Can you work these out from the model? Positions are in its coordinate system, mm. Face numbers are marked on the shaded views. A direction names the side the tool comes from. Round coordinates to 2 decimals unless told otherwise and drop trailing zeros. Loops run counter-clockwise (first coordinate to the right, second up) from the corner with the lowest first, then second, coordinate; pieces in that order, holes last. Notation, with made-up numbers: (27.5, 64) -> (54.5, 64) arc R6 ccw to (54.5, 68) -> close; hole circle Ø10 at (-24, 50). An arc over 180 degrees is marked (long way). Answer as a JSON object with one key per item and string values.
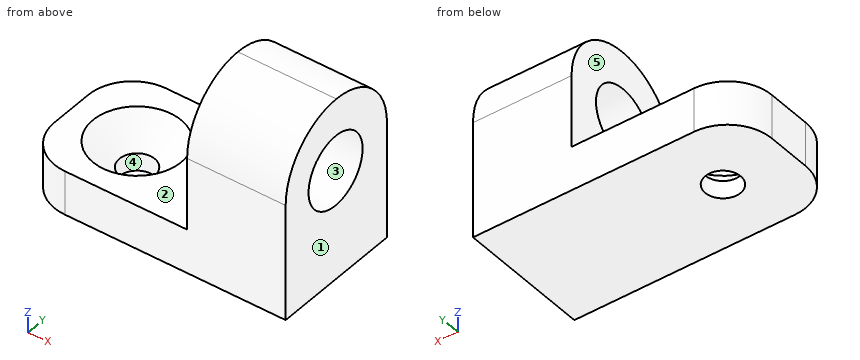
```python
from build123d import *

# Parameters (mm, degrees)
F0_W     = 18.8419777411
F0_H     = 15
F0_R     = 2
F0_W_2   = 11.1580222589
F1_DEPTH = 5
F2_SIZE  = 3
F3_DEPTH = 20.7
F4_R     = 4
F5_DEPTH = 55.3
F6_R     = 7.49999
F7_R     = 5


# Not quite as in the source:
# - a fillet or chamfer is up to 0.001 mm smaller than in the source, because OpenCascade refuses the exact size


with BuildPart() as f1:
    # F0 (on Top) → F1 (new body)
    with BuildSketch(Plane.XY):
        with Locations((9.4734227529, 0.1149109378)):
            Rectangle(F0_W, F0_H)
        with Locations((7.5819236226, 0)):
            Circle(F0_R, mode=Mode.SUBTRACT)
        with Locations((24.4734227529, 0.1149109378)):
            Rectangle(F0_W_2, F0_H)
    extrude(amount=F1_DEPTH)

    # F2
    f2_edges = [f1.edges().sort_by_distance(p)[0] for p in [
        (5.581924, 0, 5),
    ]]
    chamfer(f2_edges, length=F2_SIZE)

    # F0 (on Top) → F3 (join)
    with BuildSketch(Plane.XY):
        with Locations((24.4734227529, 0.1149109378)):
            Rectangle(F0_W_2, F0_H)
    extrude(amount=F3_DEPTH)

    # F4 (on Right) → F5 (cut)
    with BuildSketch(Plane.YZ):
        with Locations((0, 12.5060472637)):
            Circle(F4_R)
    extrude(amount=F5_DEPTH, mode=Mode.SUBTRACT)

    # F6 (radius 7.5 in the source; OpenCascade refuses exactly that, so slightly less here)
    f6_edges = [f1.edges().sort_by_distance(p)[0] for p in [
        (24.473423, -7.385089, 20.7),
        (24.473423, 7.614911, 20.7),
    ]]
    fillet(f6_edges, radius=F6_R)

    # F7
    f7_edges = [f1.edges().sort_by_distance(p)[0] for p in [
        (0.052434, -7.385089, 2.5),
        (0.052434, 7.614911, 2.5),
    ]]
    fillet(f7_edges, radius=F7_R)


solid = f1.part
```
Q1. I'm going to push a flat-ended pin straight in: pin 1 (4 mm diameter, centred on x = 17.5, y = 1, fed in from +Z). Where does the tip first touch, or does it pass through?
Determined:
{"pin 1": "z = 20.7"}
Q2. I want a section at D-D, the plane y = -6.25. Write out the boundary of the cut face in (x, z).
Determined:
{"outline": "(1.88, 0) -> (30.05, 0) -> (30.05, 17.17) -> (18.89, 17.17) -> (18.89, 5) -> (1.88, 5) -> close"}
Q3. We'd pull the mould along X, two halves only. Please class the marked faces 3, 4 and 5: pulls with the +X half, pulls with the -X half, needs draft (parallel to the pull), parting line crosses it, or undercut.
Determined:
{"face 3": "needs draft", "face 4": "undercut", "face 5": "pulls with the -X half"}
Q4. If I drill on L1, parallel to Z at x = 25.5, y = 0; L2, parallel to X at y = 4.5, z = 6.25; L3, parallel to Y at x = 27, z = 9, over which ranges is the centre line in solid material (lowest first)? Write a range as [from, to].
Determined:
{"L1": "[0, 8.51], [16.51, 20.7]", "L2": "[18.89, 30.05]", "L3": "[-7.39, -1.93], [1.93, 7.61]"}
Q5. I want a section at C-C, the plane z = 7.5. Write out the boundary of the cut face in (x, y), then the cut area to 3 significant figures.
Determined:
{"outline": "(18.89, -7.39) -> (30.05, -7.39) -> (30.05, 7.61) -> (18.89, 7.61) -> close", "area": "167 mm²"}
Q6. I want a section at B-B, the plane y = -1. Give the number of separate pieces and of enclosed holes in the cut face, then the cut area to 3 significant figures.
Determined:
{"separate pieces": "3", "enclosed holes": "0", "area": "211 mm²"}
Q7. On a 3-axis mill with a long thin cutter (end or side, diameter ignored), from which of +Z, -Z, +X, -X, +Y, -Y can I reach the whole of each face in a straight line? I mean the marked faces 1 and 2. Say none if no direction works.
Determined:
{"face 1": "+Z, -Z, +X, +Y, -Y", "face 2": "+Z, -X, +Y, -Y"}
